Print and shaded views of the part. All mm, measured from the part's lowest x, y and z. Round coordinates to 2 decimals unless told otherwise and drop trailing zeros. Write each loop counter-clockwise with the first axis right and the second up, starting at its lowest first coordinate (ties: lowest second). Pieces come first, ordered by that corner, then holes. Notation, with made-up numbers: M -5,37.5 L 5,37.5 A21 ccw 5,52.5 Z; hole C -31,35 d9. An arc over 180 degrees is marked long. Write item = value, one per line.
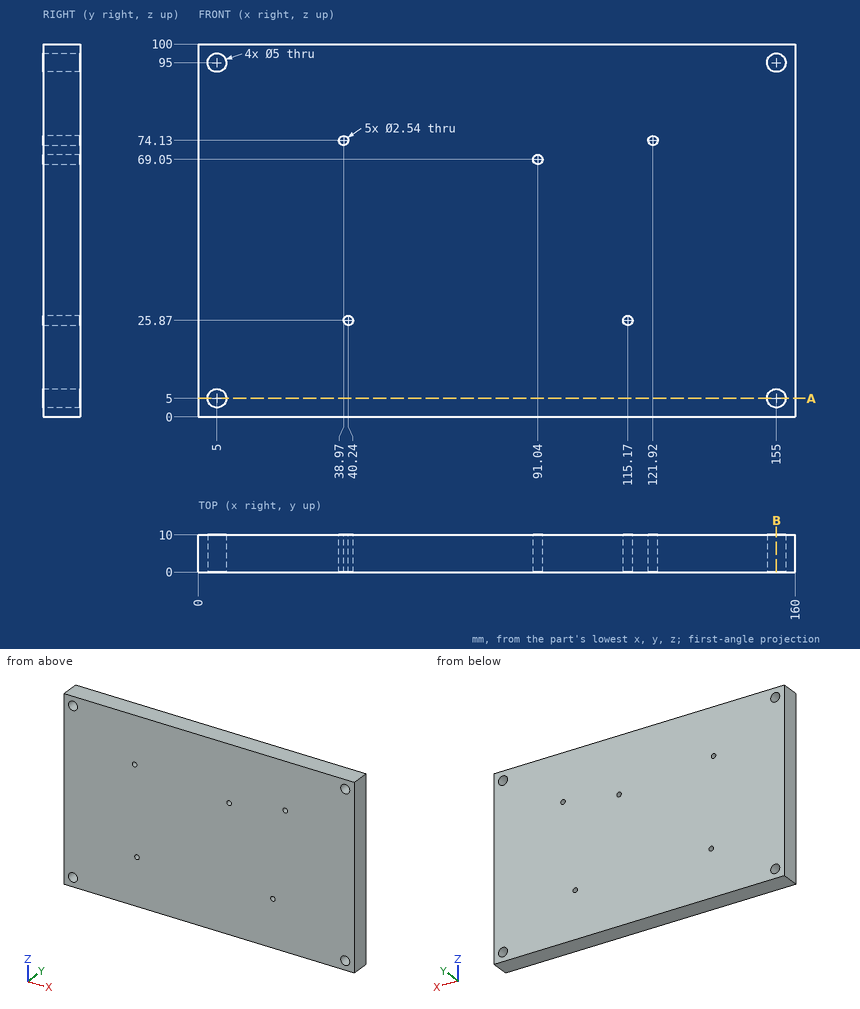
1. Band-saw the part on A-A (z = 5). List the corners of the cut face in (x, y), plus the area to 3 significant figures.
Responses:
outline = M 0,0 L 2.5,0 L 2.5,10 L 0,10 Z; M 7.5,0 L 152.5,0 L 152.5,10 L 7.5,10 Z; M 157.5,0 L 160,0 L 160,10 L 157.5,10 Z
area = 1,500 mm²
2. Probe probe 1 along X at (y, z) = (6, 95); probe 2 along X at (y, z) = (2, 25.87); probe 3 along Z at (x, y) = (122, 3.75). List the from-to ranges inside material, lowest first.
Responses:
probe_1 = 0 to 2.5, 7.5 to 152.5, 157.5 to 160
probe_2 = 0 to 38.97, 41.51 to 113.9, 116.44 to 160
probe_3 = 0 to 72.86, 75.4 to 100
3. Band-saw the part on B-B (x = 155). List the corners of the cut face in (y, z).
Responses:
outline = M 0,0 L 10,0 L 10,2.5 L 0,2.5 Z; M 0,7.5 L 10,7.5 L 10,92.5 L 0,92.5 Z; M 0,97.5 L 10,97.5 L 10,100 L 0,100 Z
